Check sheet for the modelled part. Datum: model origin and axes. Units: mm. Face numbers are marked on the shaded views. Coordinates: 2 decimals unless noted, no trailing zeros. Loops run counter-clockwise (first coordinate to the right, second up) from the corner with the lowest first, then second, coordinate; pieces in that order, holes last. Notation, with made-up numbers: (-15.5, 33.5) -> (-10.5, 33.5) arc R25 ccw to (-10.5, 66.5) -> close; hole circle Ø10 at (39, 63). An arc over 180 degrees is marked (long way). Use CSV: the item, a comma, the result in double quotes.
```python
from build123d import *

# Parameters (mm, degrees)
SKETCH1_W           = 80
SKETCH1_H           = 40
BOSS_EXTRUDE1_DEPTH = 15
SKETCH2_R           = 12
SKETCH2_R_2         = 6
CUT_EXTRUDE1_DEPTH  = 6


with BuildPart() as part:
    # Sketch1 → Boss-Extrude1 (new body)
    with BuildSketch(Plane.XY):
        Rectangle(SKETCH1_W, SKETCH1_H)
    extrude(amount=BOSS_EXTRUDE1_DEPTH)

    # Sketch2 → Cut-Extrude1 (cut)
    with BuildSketch(Plane.XY.offset(15)):
        with Locations((0, -14)):
            Circle(SKETCH2_R)
        with Locations((-13.5, -7.461651585)):
            Circle(SKETCH2_R_2)
        with Locations((-27, -14)):
            Circle(SKETCH2_R)
        with BuildLine():
            Line((-37.392304845, -20), (-16.607695155, -20))
            ThreePointArc((-16.607695155, -20), (-15.408890085, -17.105828541), (-15, -14))
            ThreePointArc((-15, -14), (-15.005629858, -13.632461014), (-15.022514151, -13.265266894))
            ThreePointArc((-15.022514151, -13.265266894), (-18.9, -10.076990951), (-18.997485849, -5.057977451))
            ThreePointArc((-18.997485849, -5.057977451), (-34.565962223, -4.685698327), (-37.392304845, -20))
        make_face()
        with BuildLine():
            ThreePointArc((10.392304845, -20), (11.591109915, -17.105828541), (12, -14))
            ThreePointArc((12, -14), (11.994370142, -13.632461014), (11.977485849, -13.265266894))
            ThreePointArc((11.977485849, -13.265266894), (8.1, -10.076990951), (8.002514151, -5.057977451))
            ThreePointArc((8.002514151, -5.057977451), (0, -2), (-8.002514151, -5.057977451))
            ThreePointArc((-8.002514151, -5.057977451), (-7.626972029, -6.233831381), (-7.5, -7.461651585))
            ThreePointArc((-7.5, -7.461651585), (-8.749469245, -11.12668331), (-11.977485849, -13.265266894))
            ThreePointArc((-11.977485849, -13.265266894), (-11.680797979, -16.749356028), (-10.392304845, -20))
            Line((-10.392304845, -20), (10.392304845, -20))
        make_face()
        with BuildLine():
            ThreePointArc((19.5, -7.461651585), (18.250530755, -11.12668331), (15.022514151, -13.265266894))
            ThreePointArc((15.022514151, -13.265266894), (15.319202021, -16.749356028), (16.607695155, -20))
            Line((16.607695155, -20), (37.392304845, -20))
            ThreePointArc((37.392304845, -20), (38.591109915, -17.105828541), (39, -14))
            ThreePointArc((39, -14), (31.897439647, -3.044860343), (18.997485849, -5.057977451))
            ThreePointArc((18.997485849, -5.057977451), (19.373027971, -6.233831381), (19.5, -7.461651585))
        make_face()
        with Locations((13.5, -7.461651585)):
            Circle(SKETCH2_R_2)
        with Locations((27, -14)):
            Circle(SKETCH2_R)
    extrude(amount=-CUT_EXTRUDE1_DEPTH, mode=Mode.SUBTRACT)


solid = part.part
```
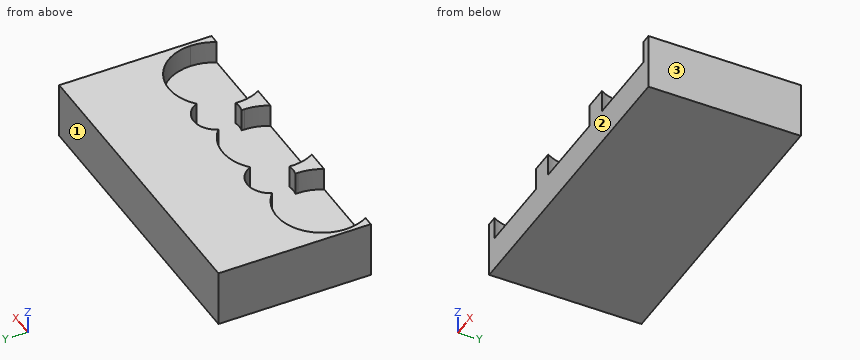
1) Thickness scan on line 1 along Z through (x, y) = (5, -17.5); line 2 along X through (y, z) = (-7.5, 10.25); line 3 along X through (y, z) = (-7, 12.5). Record the ranges inside material, lowest first. Write a range as from..to.
Answer below:
line 1,"z = 0..9"
line 2,"x = -40..-37.09, 37.09..40"
line 3,"x = -40..-36.75, 36.75..40"
2) Cross-section at B-B on x = 13. Record the boundary of the cut face in (y, z), and give its area (3 significant figures).
Answer below:
outline,"(-20, 0) -> (20, 0) -> (20, 15) -> (-1.48, 15) -> (-1.48, 9) -> (-13.44, 9) -> (-13.44, 15) -> (-20, 15) -> close"
area,"528 mm²"
3) Cross-section at C-C on y = -6. Record the boundary of the cut face in (x, z).
Answer below:
outline,"(-40, 0) -> (40, 0) -> (40, 15) -> (35.94, 15) -> (35.94, 9) -> (-35.94, 9) -> (-35.94, 15) -> (-40, 15) -> close"
4) Cross-section at D-D on x = -21. Record the boundary of the cut face in (y, z).
Answer below:
outline,"(-20, 0) -> (20, 0) -> (20, 15) -> (-3.61, 15) -> (-3.61, 9) -> (-20, 9) -> close"
5) Cross-section at A-A on z = 13.5. Record the boundary of the cut face in (x, y).
Answer below:
outline,"(-40, -20) -> (-37.39, -20) arc R12 cw to (-19, -5.06) arc R6 cw to (-8, -5.06) arc R12 cw to (8, -5.06) arc R6 cw to (19, -5.06) arc R12 cw to (37.39, -20) -> (40, -20) -> (40, 20) -> (-40, 20) -> close; (-16.61, -20) -> (-10.39, -20) arc R12 cw to (-11.98, -13.27) arc R6 cw to (-15.02, -13.27) arc R12 cw to start; (10.39, -20) -> (16.61, -20) arc R12 cw to (15.02, -13.27) arc R6 cw to (11.98, -13.27) arc R12 cw to start"
6) Go/stop test with a flat-tipped pin: pin 1 Ø4 at (x, y) = (18, -14.5) entering from +Z. Record where the tip stops, or that it passes through.
Answer below:
pin 1,"stops at z = 9"
7) Draft check along Y on the marked faces 1, 2 and 3. Enter one of: released by +Y, released by -Y, zero draft, split by the parting line, or undercut.
Answer below:
face 1,"released by +Y"
face 2,"released by -Y"
face 3,"zero draft"
